```python
from build123d import *

# Parameters (mm, degrees)
SM_BASE_FLANGE_2_DEPTH           = 0.7366
SKETCH4_R                        = 2.54
CUT_EXTRUDE_3_DEPTH              = 116.878967374
SM_EDGE_FLANGE_4_STRIP_W         = 4.4196
SM_EDGE_FLANGE_4_STRIP_H         = 0.7366
SM_EDGE_FLANGE_4_STRIP_CUT_DEPTH = 19.05
SM_EDGE_FLANGE_4_DEPTH           = 19.05
SKETCH8_W                        = 2.54
SKETCH8_H                        = 2.54
CUT_EXTRUDE_5_DEPTH              = 123.574978827
OTHER_START                      = -7.0866
OTHER_6_DEPTH                    = 0.7366


# Read off the part's stored shape, not the designer's step: 6
# Sheet-metal steps are written as plain solids
with BuildPart() as part:
    # Sketch1 → 2 (new body)
    with BuildSketch(Plane(origin=(0, 0, 0), x_dir=(1, 0, 0), z_dir=(0, 1, 0))):
        with BuildLine():
            Line((0.920589642, 0), (100.679410358, 0))
            ThreePointArc((100.679410358, 0), (101.529924286, 0.169177739), (102.250955179, 0.650955179))
            Line((102.250955179, 0.650955179), (106.029044821, 4.429044821))
            ThreePointArc((106.029044821, 4.429044821), (106.750075714, 4.910822261), (107.600589642, 5.08))
            Line((107.600589642, 5.08), (112.0775, 5.08))
            ThreePointArc((112.0775, 5.08), (113.649044821, 5.730955179), (114.3, 7.3025))
            Line((114.3, 7.3025), (114.3, 11.7475))
            ThreePointArc((114.3, 11.7475), (113.649044821, 13.319044821), (112.0775, 13.97))
            Line((112.0775, 13.97), (107.600589642, 13.97))
            ThreePointArc((107.600589642, 13.97), (106.750075714, 14.139177739), (106.029044821, 14.620955179))
            Line((106.029044821, 14.620955179), (102.250955179, 18.399044821))
            ThreePointArc((102.250955179, 18.399044821), (101.529924286, 18.880822261), (100.679410358, 19.05))
            Line((100.679410358, 19.05), (0.920589642, 19.05))
            ThreePointArc((0.920589642, 19.05), (0.070075714, 18.880822261), (-0.650955179, 18.399044821))
            Line((-0.650955179, 18.399044821), (-2.524044821, 16.525955179))
            ThreePointArc((-2.524044821, 16.525955179), (-3.245075714, 16.044177739), (-4.095589642, 15.875))
            Line((-4.095589642, 15.875), (-6.35, 15.875))
            Line((-6.35, 15.875), (-6.35, -3.175))
            Line((-6.35, -3.175), (-4.095589642, -3.175))
            ThreePointArc((-4.095589642, -3.175), (-3.245075714, -3.005822261), (-2.524044821, -2.524044821))
            Line((-2.524044821, -2.524044821), (-0.650955179, -0.650955179))
            ThreePointArc((-0.650955179, -0.650955179), (0.070075714, -0.169177739), (0.920589642, 0))
        make_face()
    extrude(amount=SM_BASE_FLANGE_2_DEPTH)

    # Sketch4 → 3 (cut, through all)
    with BuildSketch(Plane(origin=(0, 0.7366, 0), x_dir=(-1, 0, 0), z_dir=(0, 1, 0))):
        with Locations(Location((-101.6, -9.525, 0), (0, 0, 90))):
            Circle(SKETCH4_R)
    extrude(amount=-CUT_EXTRUDE_3_DEPTH, mode=Mode.SUBTRACT)

    # 4 strip (across the edge) → 4 strip cut (cut)
    with BuildSketch(Plane(origin=(-6.35, 0.7366, -15.875), x_dir=(1, 0, 0), z_dir=(0, 0, 1))):
        with Locations((-1.4732, -0.3683)):
            Rectangle(SM_EDGE_FLANGE_4_STRIP_W, SM_EDGE_FLANGE_4_STRIP_H)
    extrude(amount=SM_EDGE_FLANGE_4_STRIP_CUT_DEPTH, mode=Mode.SUBTRACT)

    # 4 section (across the edge) → 4 (add)
    with BuildSketch(Plane(origin=(-6.35, 0.7366, -15.875), x_dir=(1, 0, 0), z_dir=(0, 0, 1))):
        with BuildLine():
            Line((-0.7366, 0.7366), (-0.7366, 9.525))
            Line((-0.7366, 9.525), (0, 9.525))
            Line((0, 9.525), (0, 0.7366))
            ThreePointArc((0, 0.7366), (0.215745145, 0.215745145), (0.7366, 0))
            Line((0.7366, 0), (0.7366, -0.7366))
            ThreePointArc((0.7366, -0.7366), (-0.30510971, -0.30510971), (-0.7366, 0.7366))
        make_face()
    extrude(amount=SM_EDGE_FLANGE_4_DEPTH)

    # Sketch8 → 5 (cut, through all)
    with BuildSketch(Plane(origin=(-6.35, 0, 0), x_dir=(0, 0, -1), z_dir=(1, 0, 0))):
        with BuildLine():
            Line((-0.635, 7.7724), (-3.175, 7.7724))
            Line((-3.175, 7.7724), (-3.175, 3.9624))
            Line((-3.175, 3.9624), (-0.635, 3.9624))
            ThreePointArc((-0.635, 3.9624), (1.27, 5.8674), (-0.635, 7.7724))
        make_face()
        with Locations((6.6675, 8.9916)):
            Rectangle(SKETCH8_W, SKETCH8_H)
    extrude(amount=-CUT_EXTRUDE_5_DEPTH, mode=Mode.SUBTRACT)

    # Other 6 outline → Other 6 (cut)
    with BuildSketch(Plane.YZ.offset(OTHER_START)):
        with BuildLine():
            ThreePointArc((3.3274, 3.175), (3.776412806, 2.989012806), (3.9624, 2.54))
            Line((3.9624, 2.54), (3.9624, 3.175))
            Line((3.9624, 3.175), (3.3274, 3.175))
        make_face()
        with BuildLine():
            ThreePointArc((7.7724, 2.54), (7.958387194, 2.989012806), (8.4074, 3.175))
            Line((8.4074, 3.175), (7.7724, 3.175))
            Line((7.7724, 3.175), (7.7724, 2.54))
        make_face()
        with BuildLine():
            Line((10.2616, -5.3975), (10.2616, -4.7625))
            ThreePointArc((10.2616, -4.7625), (10.075612806, -5.211512806), (9.6266, -5.3975))
            Line((9.6266, -5.3975), (10.2616, -5.3975))
        make_face()
        with BuildLine():
            Line((10.2616, 3.175), (9.6266, 3.175))
            ThreePointArc((9.6266, 3.175), (10.075612806, 2.989012806), (10.2616, 2.54))
            Line((10.2616, 2.54), (10.2616, 3.175))
        make_face()
        with BuildLine():
            Line((10.2616, -15.875), (10.2616, -15.24))
            ThreePointArc((10.2616, -15.24), (10.075612806, -15.689012806), (9.6266, -15.875))
            Line((9.6266, -15.875), (10.2616, -15.875))
        make_face()
        with BuildLine():
            ThreePointArc((9.6266, -7.9375), (10.075612806, -8.123487194), (10.2616, -8.5725))
            Line((10.2616, -8.5725), (10.2616, -7.9375))
            Line((10.2616, -7.9375), (9.6266, -7.9375))
        make_face()
    extrude(amount=OTHER_6_DEPTH, mode=Mode.SUBTRACT)


solid = part.part
```
Read the model definition and answer for the solid it produces. Units are mm, in the model's axes. A direction names the side the tool comes from. Coordinates: 2 decimals unless noted, no trailing zeros. Loops run counter-clockwise (first coordinate to the right, second up) from the corner with the lowest first, then second, coordinate; pieces in that order, holes last.
(1) The part is cut by section A-A (z = -2.75). Determine the outline of the cut face in (x, y).
Solution:
outline: (-7.09, 1.47) arc R1.47 ccw to (-5.61, 0) - (104.35, 0) - (104.35, 0.74) - (-5.61, 0.74) arc R0.74 cw to (-6.35, 1.47) - (-6.35, 10.26) - (-7.09, 10.26) - close
(2) The part is cut by section C-C (y = 5). Determine the outline of the cut face in (x, z) (3 decimals), and give its area (3 significant figures).
Solution:
outline: (-7.087, -15.875) - (-6.35, -15.875) - (-6.35, -1.061) - (-7.087, -1.061) - close
area: 10.9 mm2
(3) Consider line 1 along X through (y, z) = (3, -12); line 2 along Y through (x, z) = (87, -18); line 3 along X through (y, z) = (0.5, -11). Determine where each line is inside the solid, lowest interval first.
Solution:
line 1: x = -7.09 to -6.35
line 2: y = 0 to 0.74
line 3: x = -6.72 to 99.53, 103.67 to 114.3
(4) The part is cut by section B-B (x = 30). Determine the outline of the cut face in (y, z).
Solution:
outline: (0, -19.05) - (0.74, -19.05) - (0.74, 0) - (0, 0) - close
(5) The mould has two halves that part along Y. Classify faces 4 (the face through (113.63, 0.36, -5.71)), 5 (the face through (54, 0.737, -8)), 6 (the face through (-6.71, 5.83, -1.27)), 7 (the face through (54, 0, -8)): released by +Y, released by -Y, zero draft, split by the parting line, or undercut.
Solution:
face 4: zero draft
face 5: released by +Y
face 6: undercut
face 7: released by -Y
(6) A tool of negligible diameter and unlimited length cuts with its end or side. For faces 1 (the face through (104.17, 0.36, -16.48)), 2 (the face through (-6.35, 6, -6)), 3 (the face through (-6.5, 4.1, -15.875)), from which of +Z, -Z, +X, -X, +Y, -Y can it reach the whole face along a straight path? Write none if from no direction.
Solution:
face 1: -Z, +X, +Y, -Y
face 2: +Z, -Z, +X, +Y
face 3: -Z, -X, +Y, -Y
(7) Flat-ended cylindrical pins translate along their axes: pin 1 Ø3.5 at (x, y) = (-5, 5) entering from -Z (3 decimals); pin 2 Ø0.8 at (x, y) = (110.5, 0) entering from +Z; pin 3 Ø5 at (x, y) = (69, 1.5) entering from +Z. Find the tip coordinate at first contact, or state that the pin passes through.
Solution:
pin 1: stops at z = -15.875
pin 2: stops at z = -5.08
pin 3: stops at z = 0
